Geometry check sheet. Reference: drawing and pictorial views, mm from the part's lowest x, y, z. A direction names the side the tool comes from. Round coordinates to 2 decimals unless told otherwise and drop trailing zeros. Loops run counter-clockwise (first coordinate to the right, second up) from the corner with the lowest first, then second, coordinate; pieces in that order, holes last. Notation, with made-up numbers: (70, 13) - (92, 13) arc R20 ccw to (92, 18) - close; hole circle Ø5 at (40, -4.5). An arc over 180 degrees is marked (long way). Put each result on its own line as item: value. Start each with the question number.
Item 1: Material ranges on line 1 along X through (y, z) = (47.5, 6.5); line 2 along Y through (x, z) = (119, 13.25) (1 decimal); line 3 along Y through (x, z) = (33, 2.5), recorded low to high.
Item 2: Section check A-A, the plane z = 4.25. Give the number of separate pieces and of enclosed holes in the cut face, and give its area (3 significant figures).
Item 3: Section check B-B, the plane y = 58. Record the cut outline in (x, z).
Item 4: Section check D-D, the plane x = 176.5. Record the cut outline in (y, z).
Item 5: Tool access check on the marked faces 1 and 2. Record the directions out of +Z, -Z, +X, -X, +Y, -Y that give a thin tool (end or side, any length) a straight path to the whole face; none if there is none.
Item 6: Section check C-C, the plane x = 80. Record the cut outline in (y, z) (1 decimal).
Item 7: Draft check along Y on the marked faces 3, 4 and 5. Enter one of: pulls with the +Y half, pulls with the -Y half, needs draft (parallel to the pull), parting line crosses it, or undercut.
Item 8: Gauge pin test, flat ends, axial feed: pin 1 Ø1.5 at (y, z) = (17.5, 16.5) entering from -X (1 decimal); pin 2 Ø5.5 at (x, z) = (31.5, 13) entering from -Y; pin 3 Ø6 at (y, z) = (13.5, 9) entering from +X. Record the tip position at first contact, or that the pin passes through.
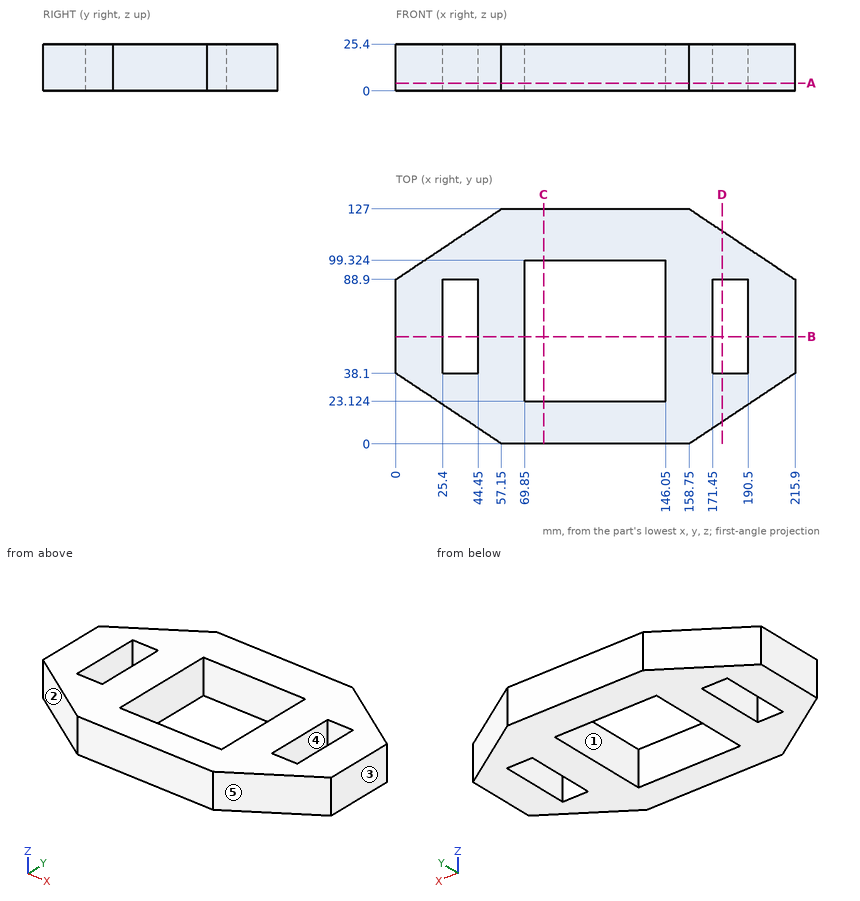
Check result:
1. line 1: 0 to 25.4, 44.45 to 69.85, 146.05 to 171.45, 190.5 to 215.9
1. line 2: 0 to 23.1, 99.3 to 127
1. line 3: 16.1 to 38.1, 88.9 to 110.9
2. separate pieces: 1
2. enclosed holes: 3
2. area: 15,300 mm²
3. outline: (0, 0) - (25.4, 0) - (25.4, 25.4) - (0, 25.4) - close; (44.45, 0) - (69.85, 0) - (69.85, 25.4) - (44.45, 25.4) - close; (146.05, 0) - (171.45, 0) - (171.45, 25.4) - (146.05, 25.4) - close; (190.5, 0) - (215.9, 0) - (215.9, 25.4) - (190.5, 25.4) - close
4. outline: (11.83, 0) - (38.1, 0) - (38.1, 25.4) - (11.83, 25.4) - close; (88.9, 0) - (115.17, 0) - (115.17, 25.4) - (88.9, 25.4) - close
5. face 1: +Z, -Z
5. face 2: +Z, -Z, -X, -Y
6. outline: (0, 0) - (23.1, 0) - (23.1, 25.4) - (0, 25.4) - close; (99.3, 0) - (127, 0) - (127, 25.4) - (99.3, 25.4) - close
7. face 3: needs draft
7. face 4: undercut
7. face 5: pulls with the -Y half
8. pin 1: x = 29.8
8. pin 2: y = 15.27
8. pin 3: x = 183.5
